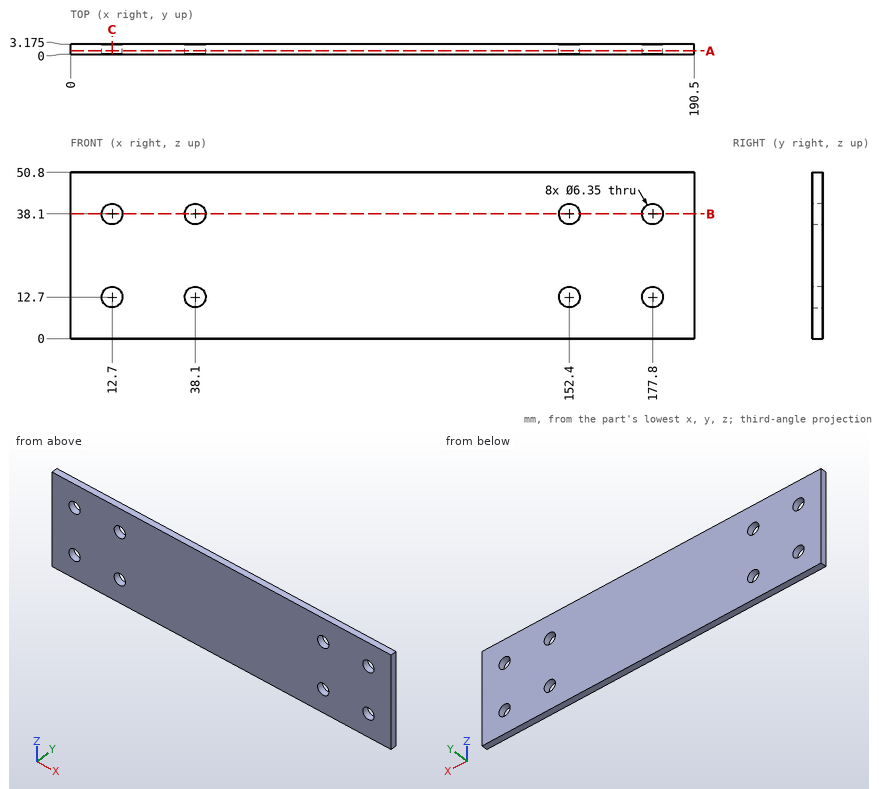
Study the drawing (mm; zero at the part's minimum x, y, z) and answer. Give positions to 0.01 mm unless a question says otherwise; leave off trailing zeros. Order: outer loops, then holes, each group sorted by start corner. A loop starts at its lowest first (then second) coordinate and runs counter-clockwise, first axis right, second up. Notation, with made-up numbers: (-39, 48) -> (-33, 48) arc R26 ccw to (-33, 66) -> close; hole circle Ø8 at (86.5, -30.5). An arc over 180 degrees is marked (long way). Put each result on its own line as item: value.
Item 1: Straight lines are drawn through the part: line 1 (X direction, y = 0.75, z = 12.7) (3 decimals); line 2 (Z direction, x = 177.8, y = 2.3) (3 decimals); line 3 (X direction, y = 2.7, z = 10). For each, find the intervals that lie inside material, in ascending order.
Established:
line 1: x = 0 to 9.525, 15.875 to 34.925, 41.275 to 149.225, 155.575 to 174.625, 180.975 to 190.5
line 2: z = 0 to 9.525, 15.875 to 34.925, 41.275 to 50.8
line 3: x = 0 to 11.03, 14.37 to 36.43, 39.77 to 150.73, 154.07 to 176.13, 179.47 to 190.5
Item 2: A cutting plane is placed at B-B on z = 38.1. Give the vertices of the cut face in (x, y) (3 decimals), plus the area to 3 significant figures.
Established:
outline: (0, 0) -> (9.525, 0) -> (9.525, 3.175) -> (0, 3.175) -> close; (15.875, 0) -> (34.925, 0) -> (34.925, 3.175) -> (15.875, 3.175) -> close; (41.275, 0) -> (149.225, 0) -> (149.225, 3.175) -> (41.275, 3.175) -> close; (155.575, 0) -> (174.625, 0) -> (174.625, 3.175) -> (155.575, 3.175) -> close; (180.975, 0) -> (190.5, 0) -> (190.5, 3.175) -> (180.975, 3.175) -> close
area: 524 mm^2
Item 3: A cutting plane is placed at A-A on y = 1.1. Count the separate pieces of the cut face and the enclosed holes in it, plus the area to 3 significant figures.
Established:
separate pieces: 1
enclosed holes: 8
area: 9,420 mm^2
Item 4: A cutting plane is placed at C-C on x = 12.7. Give the vertices of the cut face in (y, z) (3 decimals), plus the area to 3 significant figures.
Established:
outline: (0, 0) -> (3.175, 0) -> (3.175, 9.525) -> (0, 9.525) -> close; (0, 15.875) -> (3.175, 15.875) -> (3.175, 34.925) -> (0, 34.925) -> close; (0, 41.275) -> (3.175, 41.275) -> (3.175, 50.8) -> (0, 50.8) -> close
area: 121 mm^2
Item 5: Given P1, Ø7.5, axis at x = 12.7, z = 38.1, coming from the -Y side; P2, Ø5, axis at x = 38.1, z = 12.7, coming from the -Y side, each flat-ended and moving along its own axis, determine where each tip first touches the part or whether it passes through.
Established:
P1: stops at y = 0
P2: passes through
